```python
from build123d import *

# Parameters (mm, degrees)
SKIZZE1_W                       = 58
SKIZZE1_H                       = 12.7
SKIZZE1_R                       = 2
AUFSATZ_LINEAR_AUSTRAGEN1_DEPTH = 12.7
SKIZZE2_R                       = 5
SCHNITT_LINEAR_AUSTRAGEN1_DEPTH = 12.7


with BuildPart() as part:
    # Skizze1 → Aufsatz-Linear austragen1 (new body)
    with BuildSketch(Plane(origin=(0, 0, 0), x_dir=(1, 0, 0), z_dir=(0, 1, 0))):
        Rectangle(SKIZZE1_W, SKIZZE1_H)
        with Locations(Location((-24.5, 0, 0), (0, 0, 270))):
            Circle(SKIZZE1_R, mode=Mode.SUBTRACT)
        with Locations(Location((-17, 0, 0), (0, 0, 270))):
            Circle(SKIZZE1_R, mode=Mode.SUBTRACT)
        with Locations(Location((24.5, 0, 0), (0, 0, 270))):
            Circle(SKIZZE1_R, mode=Mode.SUBTRACT)
        with Locations(Location((17, 0, 0), (0, 0, 270))):
            Circle(SKIZZE1_R, mode=Mode.SUBTRACT)
    extrude(amount=AUFSATZ_LINEAR_AUSTRAGEN1_DEPTH)

    # Skizze2 → Schnitt-Linear austragen1 (cut)
    with BuildSketch(Plane.XY.offset(6.35)):
        with Locations((-4, 6.35)):
            Circle(SKIZZE2_R)
        with Locations((4, 6.35)):
            Circle(SKIZZE2_R)
    extrude(amount=-SCHNITT_LINEAR_AUSTRAGEN1_DEPTH, mode=Mode.SUBTRACT)


solid = part.part
```
The model under review builds one solid part; all positions refer to its coordinate system, in mm. Coordinates: 2 decimals unless noted, no trailing zeros. Write each loop counter-clockwise with the first axis right and the second up, starting at its lowest first coordinate (ties: lowest second). Pieces come first, ordered by that corner, then holes. Notation, with made-up numbers: (-5.5, 57.5) - (1.5, 57.5) arc R7 ccw to (1.5, 69.5) - close; hole circle Ø7 at (30, 58.5). An arc over 180 degrees is marked (long way). Write item = value, one per line.
(1) For P1, Ø6.5, axis at x = -17, z = 0, coming from the -Y side, flat-tipped, find the tip position at first contact; note if it passes through.
Result sheet:
P1 = 0
(2) For line 1 (X direction, y = 6.25, z = 0); line 2 (X direction, y = 6.35, z = -1); line 3 (X direction, y = 6.25, z = 2.5), list the stretches that pass through material, from the lowest coordinate up. Write a range as [from, to].
Result sheet:
line_1 = [-29, -26.5], [-22.5, -19], [-15, -9], [9, 15], [19, 22.5], [26.5, 29]
line_2 = [-29, -26.23], [-22.77, -18.73], [-15.27, -9], [9, 15.27], [18.73, 22.77], [26.23, 29]
line_3 = [-29, -9], [9, 29]
(3) Mouldability with a two-part tool opening along Z and no side actions: class faces 1 (the face through (-25.7, 6.3, -1.6)), 2 (the face through (-15, 6, 0)), 3 (the face through (0, 10, -6.35)), 4 (the face through (0, 0, 0)) as pulls with the +Z half, pulls with the -Z half, needs draft (parallel to the pull), parting line crosses it, or undercut.
Result sheet:
face_1 = undercut
face_2 = undercut
face_3 = pulls with the -Z half
face_4 = needs draft
(4) Consider section A-A, the plane y = 6.35. Give the boundary of the cut face in (x, z), then the cut area to 3 significant figures.
Result sheet:
outline = (-29, -6.35) - (-9, -6.35) - (-9, 6.35) - (-29, 6.35) - close; (9, -6.35) - (29, -6.35) - (29, 6.35) - (9, 6.35) - close; hole circle Ø4 at (-24.5, 0); hole circle Ø4 at (-17, 0); hole circle Ø4 at (17, 0); hole circle Ø4 at (24.5, 0)
area = 458 mm^2
(5) Consider section D-D, the plane y = 10.5. Give the boundary of the cut face in (x, z), then the cut area to 3 significant figures.
Result sheet:
outline = (-29, -6.35) - (-6.79, -6.35) - (-6.79, 6.35) - (-29, 6.35) - close; (-1.21, -6.35) - (1.21, -6.35) - (1.21, 6.35) - (-1.21, 6.35) - close; (6.79, -6.35) - (29, -6.35) - (29, 6.35) - (6.79, 6.35) - close; hole circle Ø4 at (-24.5, 0); hole circle Ø4 at (-17, 0); hole circle Ø4 at (17, 0); hole circle Ø4 at (24.5, 0)
area = 545 mm^2
(6) Consider section B-B, the plane z = -1.5. Give the boundary of the cut face in (x, y), then the cut area to 3 significant figures.
Result sheet:
outline = (-29, 0) - (-25.82, 0) - (-25.82, 12.7) - (-29, 12.7) - close; (-23.18, 0) - (-18.32, 0) - (-18.32, 12.7) - (-23.18, 12.7) - close; (-15.68, 0) - (15.68, 0) - (15.68, 12.7) - (-15.68, 12.7) - close; (18.32, 0) - (23.18, 0) - (23.18, 12.7) - (18.32, 12.7) - close; (25.82, 0) - (29, 0) - (29, 12.7) - (25.82, 12.7) - close; hole (0, 3.35) arc R5 ccw (long way) to (0, 9.35) arc R5 ccw (long way) to start
area = 453 mm^2
(7) Consider section C-C, the plane x = -4. Give the boundary of the cut face in (y, z), then the cut area to 3 significant figures.
Result sheet:
outline = (0, -6.35) - (1.35, -6.35) - (1.35, 6.35) - (0, 6.35) - close; (11.35, -6.35) - (12.7, -6.35) - (12.7, 6.35) - (11.35, 6.35) - close
area = 34.3 mm^2
